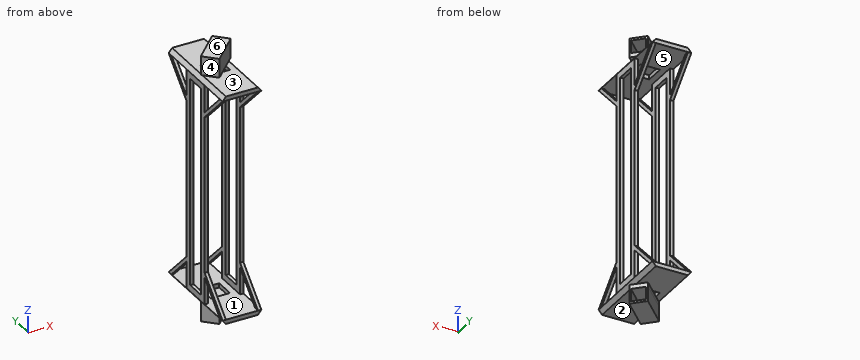
```python
from build123d import *

# Parameters (mm, degrees)
SKETCH1_W             = 38.1
SKETCH1_H             = 38.1
BOSS_EXTRUDE1_DEPTH   = 5.08
SKETCH2_W             = 4
SKETCH2_H             = 38.1
BOSS_EXTRUDE2_DEPTH   = 263.31036223
BOSS_EXTRUDE2_2_DEPTH = 263.31036223
BOSS_EXTRUDE4_DEPTH   = 38.1
SKETCH5_W             = 22.86
SKETCH5_H             = 22.86
CUT_EXTRUDE1_DEPTH    = 354.24236223
SKETCH6_W             = 248.07036223
SKETCH6_H             = 22.86
CUT_EXTRUDE2_DEPTH    = 354.24236223
BOSS_EXTRUDE5_DEPTH   = 38.1
BOSS_EXTRUDE6_DEPTH   = 4
MIRROR9_COPY_1_DEPTH  = 4
BOSS_EXTRUDE8_DEPTH   = 5.08
BOSS_EXTRUDE9_DEPTH   = 15
BOSS_EXTRUDE10_DEPTH  = 2.54


with BuildPart() as part:
    # Sketch1 → Boss-Extrude1 (new body)
    with BuildSketch(Plane.XY):
        Rectangle(SKETCH1_W, SKETCH1_H)
    extrude(amount=BOSS_EXTRUDE1_DEPTH)



with BuildPart() as body_2:
    # Sketch2 → Boss-Extrude2 (new body)
    with BuildSketch(Plane(origin=(0, 0, 0), x_dir=(-1, 0, 0), z_dir=(0, 0, -1))):
        with Locations((21.05, 0)):
            Rectangle(SKETCH2_W, SKETCH2_H)
    extrude(amount=BOSS_EXTRUDE2_DEPTH)


with BuildPart() as body_3:
    # Sketch2 → Boss-Extrude2 2 (new body)
    with BuildSketch(Plane(origin=(0, 0, 0), x_dir=(-1, 0, 0), z_dir=(0, 0, -1))):
        with Locations((-21.05, 0)):
            Rectangle(SKETCH2_W, SKETCH2_H)
    extrude(amount=BOSS_EXTRUDE2_2_DEPTH)


with BuildPart() as part_1:
    add(part.part)

    add(body_2.part)  # Boss-Extrude4 merges body 2

    add(body_3.part)  # Boss-Extrude4 merges body 3
    # Sketch4 → Boss-Extrude4 (add)
    with BuildSketch(Plane(origin=(0, 19.05, 0), x_dir=(1, 0, 0), z_dir=(0, 1, 0))):
        Polygon((23.05, 0), (19.05, -5.08), (19.05, 0), align=None)
        Polygon((-19.05, 0), (-19.05, -5.08), (-23.05, 0), align=None)
    extrude(amount=-BOSS_EXTRUDE4_DEPTH)

    # Mirror2: part across plane


with BuildPart() as part_2:
    add(part_1.part)
    add(part_1.part.mirror(Plane(origin=(0, 0, -131.655181115), x_dir=(1, 0, 0), z_dir=(0, 0, -1))))

    # Sketch5 → Cut-Extrude1 (cut)
    with BuildSketch(Plane.XY.offset(5.08)):
        Rectangle(SKETCH5_W, SKETCH5_H)
    extrude(amount=-CUT_EXTRUDE1_DEPTH, mode=Mode.SUBTRACT)

    # Sketch6 → Cut-Extrude2 (cut)
    with BuildSketch(Plane.ZY.offset(23.05)):
        with Locations((-131.655181115, 0)):
            Rectangle(SKETCH6_W, SKETCH6_H)
    extrude(amount=-CUT_EXTRUDE2_DEPTH, mode=Mode.SUBTRACT)

    # Sketch7 → Boss-Extrude5 (add)
    with BuildSketch(Plane(origin=(0, 19.05, 0), x_dir=(1, 0, 0), z_dir=(0, 1, 0))):
        Polygon((-19.05, 0), (-23.05, 0), (-19.05, -5.08), (19.05, -5.08), (23.05, 0), (19.05, 0), align=None)
        Polygon((19.05, 268.39036223), (23.05, 263.31036223), (19.05, 263.31036223), (-19.05, 263.31036223), (-23.05, 263.31036223), (-19.05, 268.39036223), align=None)
    boss_extrude5 = extrude(amount=BOSS_EXTRUDE5_DEPTH)

    # Sketch8 → Boss-Extrude6 (add)
    with BuildSketch(Plane.ZY.offset(23.05)):
        Polygon((0, 57.15), (-38.1, 19.05), (-32.395584898, 19.05), (0, 51.445584898), align=None)
        Polygon((-230.914777332, 19.05), (-263.31036223, 51.445584898), (-263.31036223, 57.15), (-225.21036223, 19.05), align=None)
    boss_extrude6 = extrude(amount=-BOSS_EXTRUDE6_DEPTH)

    # Mirror8: Boss-Extrude6 across plane
    add(boss_extrude6.mirror(Plane(origin=(0, 0, 0), x_dir=(0, 0, 1), z_dir=(1, 0, 0))))

    # Mirror9: Boss-Extrude5, Boss-Extrude6 across plane
    add(boss_extrude5.mirror(Plane.ZX))
    add(boss_extrude6.mirror(Plane.ZX))

    # Mirror9 copy 1 sketch → Mirror9 copy 1 (add)
    with BuildSketch(Plane(origin=(23.05, 0, 0), x_dir=(0, 0, 1), z_dir=(1, 0, 0))):
        Polygon((0, 57.15), (-38.1, 19.05), (-32.395584898, 19.05), (0, 51.445584898), align=None)
        Polygon((-230.914777332, 19.05), (-263.31036223, 51.445584898), (-263.31036223, 57.15), (-225.21036223, 19.05), align=None)
    extrude(amount=-MIRROR9_COPY_1_DEPTH)

    # Sketch11 → Boss-Extrude8 (add)
    with BuildSketch(Plane.XY.offset(5.08)):
        Polygon((-18.529352083, -7.922750365), (-7.922750365, -18.529352083), (-6.126699141, -20.325403307), (24.406171671, 10.207467504), (10.207467504, 24.406171671), (8.41141628, 22.610120446), (-20.325403307, -6.126699141), align=None)
    boss_extrude8 = extrude(amount=BOSS_EXTRUDE8_DEPTH)

    # Sketch12 → Boss-Extrude9 (add)
    with BuildSketch(Plane.XY.offset(10.16)):
        Polygon((24.406171671, 10.207467504), (-6.126699141, -20.325403307), (-20.325403307, -6.126699141), (10.207467504, 24.406171671), (11.477467504, 23.136171671), (10.207467504, 21.866171671), (-17.785403307, -6.126699141), (-6.126699141, -17.785403307), (21.866171671, 10.207467504), (23.136171671, 11.477467504), align=None)
    boss_extrude9 = extrude(amount=BOSS_EXTRUDE9_DEPTH)

    # Sketch13 → Boss-Extrude10 (add)
    with BuildSketch(Plane.XY.offset(25.16)):
        Polygon((-20.325403307, -6.126699141), (10.207467504, 24.406171671), (24.406171671, 10.207467504), (-6.126699141, -20.325403307), align=None)
    boss_extrude10 = extrude(amount=BOSS_EXTRUDE10_DEPTH)

    # Mirror12: Boss-Extrude8, Boss-Extrude9, Boss-Extrude10 across plane
    add(boss_extrude8.mirror(Plane(origin=(0, 0, -131.655181115), x_dir=(1, 0, 0), z_dir=(0, 0, -1))))
    add(boss_extrude9.mirror(Plane(origin=(0, 0, -131.655181115), x_dir=(1, 0, 0), z_dir=(0, 0, -1))))
    add(boss_extrude10.mirror(Plane(origin=(0, 0, -131.655181115), x_dir=(1, 0, 0), z_dir=(0, 0, -1))))


solid = part_2.part
```
CAD build for the part. Positions are in the model's coordinates, mm. Face numbers are marked on the shaded views. A direction names the side the tool comes from. Round coordinates to 2 decimals unless told otherwise and drop trailing zeros. Write each loop counter-clockwise with the first axis right and the second up, starting at its lowest first coordinate (ties: lowest second). Pieces come first, ordered by that corner, then holes. Notation, with made-up numbers: (-27.5, 41.5) - (-9.5, 41.5) arc R24 cw to (-9.5, 65.5) - close; hole circle Ø4 at (79.5, -26). An arc over 180 degrees is marked (long way). Return JSON: item names as keys, results as strings. Group by question number.
Item 1: Band-saw the part on B-B on y = 32.5. List the corners of the cut face in (x, z).
Item 2: 3-axis set-ups, long thin cutter, end or side, ignore diameter. For the marked faces 4, 5 and 6: which of +Z, -Z, +X, -X, +Y, -Y reach the whole face in a straight line?
Item 3: Probe probe 1 along Z at (x, y) = (10.5, -29.5); probe 2 along X at (y, z) = (-4, -4); probe 3 along Z at (x, y) = (21, 36). List the from-to ranges inside material, lowest first.
Item 4: Mould opens along Z. For the marked faces 1, 2 and 3 say: +Z half, -Z half, draft (parallel to the pull), parting line (faces both ways), or undercut.
Item 5: Band-saw the part on C-C on z = -243.5. State how many separate pieces and enclosed holes the cut face has, plus the area to 3 significant figures.
Item 6: Band-saw the part on A-A on z = -128. List the corners of the cut face in (x, y).
Item 7: Band-saw the part on D-D on x = 16. List the corners of the cut face in (y, z), plus the area to 3 significant figures.
Item 8: Flat gauge pins, fed straight in: pin 1 Ø1.5 at (y, z) = (-1.5, -266.5) entering from +X; pin 2 Ø4 at (x, y) = (14, -27) entering from -Z; pin 3 Ø2 at (x, z) = (-21.5, -24) entering from -Y. Where does each tip first touch, or does it go through?
Resolved:
{
 "1": {"outline": "(-23.05, -263.31) - (-19.05, -268.39) - (19.05, -268.39) - (23.05, -263.31) - close; (-23.05, -244.36) - (-19.05, -244.36) - (-19.05, -238.66) - (-23.05, -238.66) - close; (-23.05, -24.65) - (-19.05, -24.65) - (-19.05, -18.95) - (-23.05, -18.95) - close; (-23.05, 0) - (23.05, 0) - (19.05, 5.08) - (-19.05, 5.08) - close; (19.05, -244.36) - (23.05, -244.36) - (23.05, -238.66) - (19.05, -238.66) - close; (19.05, -24.65) - (23.05, -24.65) - (23.05, -18.95) - (19.05, -18.95) - close"},
 "2": {"face 4": "+Z, -X, -Y", "face 5": "none", "face 6": "+Z, +X, -X, +Y, -Y"},
 "3": {"probe 1": "z = -268.39 to -263.31, 0 to 5.08", "probe 2": "x = -23.05 to -19.05, 19.05 to 23.05", "probe 3": "z = -265.91 to -263.31, -247.86 to -242.16, -21.15 to -15.45, 0 to 2.6"},
 "4": {"face 1": "undercut", "face 2": "-Z half", "face 3": "+Z half"},
 "5": {"separate pieces": "8", "enclosed holes": "0", "area": "213 mm²"},
 "6": {"outline": "(-23.05, -19.05) - (-19.05, -19.05) - (-19.05, -11.43) - (-23.05, -11.43) - close; (-23.05, 11.43) - (-19.05, 11.43) - (-19.05, 19.05) - (-23.05, 19.05) - close; (19.05, -19.05) - (23.05, -19.05) - (23.05, -11.43) - (19.05, -11.43) - close; (19.05, 11.43) - (23.05, 11.43) - (23.05, 19.05) - (19.05, 19.05) - close"},
 "7": {"outline": "(-57.15, -268.39) - (1.8, -268.39) - (1.8, -291.01) - (18.61, -291.01) - (18.61, -288.47) - (4.34, -288.47) - (4.34, -273.47) - (18.61, -273.47) - (18.61, -268.39) - (57.15, -268.39) - (57.15, -263.31) - (-57.15, -263.31) - close; (-57.15, 0) - (57.15, 0) - (57.15, 5.08) - (18.61, 5.08) - (18.61, 10.16) - (4.34, 10.16) - (4.34, 25.16) - (18.61, 25.16) - (18.61, 27.7) - (1.8, 27.7) - (1.8, 5.08) - (-57.15, 5.08) - close", "area": "1,490 mm²"},
 "8": {"pin 1": "stops at x = 21.13", "pin 2": "stops at z = -268.39", "pin 3": "stops at y = -34.15"}
}
